The model under review builds one solid part; all positions refer to its coordinate system, in mm. A direction names the side the tool comes from. Give positions to 0.01 mm unless a question says otherwise; leave off trailing zeros. Loops run counter-clockwise (first coordinate to the right, second up) from the corner with the lowest first, then second, coordinate; pieces in that order, holes last. Notation, with made-up numbers: M 88.25,16.25 L 115.25,16.25 A21 ccw 115.25,36.25 Z; hole C 62.5,-14.5 d5. An arc over 180 degrees is marked long. Put each result on its own line as item: value. Start each with the question number.
```python
from build123d import *

# Parameters (mm, degrees)
SKETCH_1_R               = 6
SKETCH_1_R_2             = 4
EXTRUDE_1_DEPTH          = 5
CUT_EXTRUDE_1_REACH      = 16.318
CUT_EXTRUDE_1_END_RADIUS = 4
SKETCH_2_R               = 1.45
SKETCH_3_W               = 30
SKETCH_3_H               = 31
SKETCH_3_R               = 6
EXTRUDE_1_2_DEPTH        = 2
SKETCH_6_W               = 2
SKETCH_6_H               = 4
EXTRUDE_2_DEPTH          = 12
EXTRUDE_3_DEPTH          = 1.5
EXTRUDE_START            = -1.25
EXTRUDE_4_DEPTH          = 1.5
CUT_EXTRUDE_3_REACH      = 30.745
SKETCH_11_R              = 0.95
CUT_EXTRUDE_4_REACH      = 30.745
SKETCH_12_R              = 0.95
CUT_EXTRUDE_5_REACH      = 26.683
SKETCH_14_W              = 2
SKETCH_14_H              = 12
CUT_EXTRUDE_6_DEPTH      = 0.3
SKETCH_15_W              = 2
SKETCH_15_H              = 12
CUT_EXTRUDE_7_DEPTH      = 0.3


with BuildPart() as part:
    # 草图1 → Extrude 1 (new body)
    with BuildSketch(Plane(origin=(0, 0, 0), x_dir=(1, 0, 0), z_dir=(0, 1, 0))):
        Circle(SKETCH_1_R)
        Circle(SKETCH_1_R_2, mode=Mode.SUBTRACT)
    extrude(amount=EXTRUDE_1_DEPTH)

    # 切除-拉伸1: up to this cylinder (the profile starts outside it)
    cut_extrude_1_end = Plane(origin=(0, 2.637062, 0), z_dir=(0, -1, 0)) * Cylinder(CUT_EXTRUDE_1_END_RADIUS, 41.636, mode=Mode.PRIVATE)
    # 草图2 → 切除-拉伸1 (cut, up to the surface)
    with BuildSketch(Plane(origin=(6, 0, 0), x_dir=(0, 0, -1), z_dir=(1, 0, 0)), mode=Mode.PRIVATE) as cut_extrude_1_sk1:
        with Locations((0, 2.637062232)):
            Circle(SKETCH_2_R)
    cut_extrude_1_tool1 = extrude(cut_extrude_1_sk1.sketch, amount=-CUT_EXTRUDE_1_REACH, mode=Mode.PRIVATE) - cut_extrude_1_end
    add(cut_extrude_1_tool1.solids().sort_by_distance((6, 2.637062, 0))[0], mode=Mode.SUBTRACT)

    # 草图3 → Extrude 1 2 (add)
    # profile 1 of 2: a face of its own
    with BuildSketch(Plane(origin=(0, 5, 0), x_dir=(1, 0, 0), z_dir=(0, 1, 0))):
        Rectangle(SKETCH_3_W, SKETCH_3_H)
        Circle(SKETCH_3_R, mode=Mode.SUBTRACT)
    # profile 2 of 2: a face of its own
    with BuildSketch(Plane(origin=(0, 5, 0), x_dir=(1, 0, 0), z_dir=(0, 1, 0))):
        Circle(SKETCH_3_R)
    extrude(amount=EXTRUDE_1_2_DEPTH)

    # 草图6 → 凸台-拉伸2 (add)
    with BuildSketch(Plane(origin=(0, 7, 0), x_dir=(1, 0, 0), z_dir=(0, 1, 0))):
        with Locations((-1, 13.5)):
            Rectangle(SKETCH_6_W, SKETCH_6_H)
        with Locations((-1, -13.5)):
            Rectangle(SKETCH_6_W, SKETCH_6_H)
    extrude(amount=EXTRUDE_2_DEPTH)

    # 草图9 → 凸台-拉伸3 (add)
    with BuildSketch(Plane.XY.offset(-12.75)):
        Polygon((-2, 7), (-8, 7), (-2, 17), align=None)
    extrude(amount=-EXTRUDE_3_DEPTH)

    # 草图10 → 凸台-拉伸4 (add)
    with BuildSketch(Plane.XY.offset(15.5).offset(EXTRUDE_START)):
        Polygon((-2, 7), (-2, 17), (-8, 7), align=None)
    extrude(amount=-EXTRUDE_4_DEPTH)

    # 草图11 → 切除-拉伸3 (cut, up to next)
    with BuildSketch(Plane(origin=(0, 0, 0), x_dir=(0, 0, -1), z_dir=(1, 0, 0)), mode=Mode.PRIVATE) as cut_extrude_3_sk1:
        with Locations((-13.5, 13)):
            Circle(SKETCH_11_R)
    cut_extrude_3_tool1 = extrude(cut_extrude_3_sk1.sketch, amount=-CUT_EXTRUDE_3_REACH, mode=Mode.PRIVATE) & part.part
    add(cut_extrude_3_tool1.solids().sort_by_distance((0, 13, 13.5))[0], mode=Mode.SUBTRACT)

    # 草图12 → 切除-拉伸4 (cut, up to next)
    with BuildSketch(Plane(origin=(0, 0, 0), x_dir=(0, 0, -1), z_dir=(1, 0, 0)), mode=Mode.PRIVATE) as cut_extrude_4_sk1:
        with Locations((13.5, 13)):
            Circle(SKETCH_12_R)
    cut_extrude_4_tool1 = extrude(cut_extrude_4_sk1.sketch, amount=-CUT_EXTRUDE_4_REACH, mode=Mode.PRIVATE) & part.part
    add(cut_extrude_4_tool1.solids().sort_by_distance((0, 13, -13.5))[0], mode=Mode.SUBTRACT)

    # 草图13 → 切除-拉伸5 (cut, up to next)
    with BuildSketch(Plane(origin=(0, 7, 0), x_dir=(1, 0, 0), z_dir=(0, 1, 0)), mode=Mode.PRIVATE) as cut_extrude_5_sk1:
        with BuildLine():
            ThreePointArc((-5.178078794, -15.5), (-6.61861505, -14.941768129), (-8, -14.25))
            ThreePointArc((-8, -14.25), (-12.137612149, -10.942617206), (-15, -6.485560886))
            Line((-15, -6.485560886), (-15, -15.5))
            Line((-15, -15.5), (-5.178078794, -15.5))
        make_face()
    cut_extrude_5_tool1 = extrude(cut_extrude_5_sk1.sketch, amount=-CUT_EXTRUDE_5_REACH, mode=Mode.PRIVATE) & part.part
    # 草图13 → 切除-拉伸5 (cut, up to next)
    with BuildSketch(Plane(origin=(0, 7, 0), x_dir=(1, 0, 0), z_dir=(0, 1, 0)), mode=Mode.PRIVATE) as cut_extrude_5_sk2:
        with BuildLine():
            ThreePointArc((15, -6.485560886), (11.050056294, -12.039881889), (5.178078794, -15.5))
            Line((5.178078794, -15.5), (15, -15.5))
            Line((15, -15.5), (15, -6.485560886))
        make_face()
    cut_extrude_5_tool2 = extrude(cut_extrude_5_sk2.sketch, amount=-CUT_EXTRUDE_5_REACH, mode=Mode.PRIVATE) & part.part
    # 草图13 → 切除-拉伸5 (cut, up to next)
    with BuildSketch(Plane(origin=(0, 7, 0), x_dir=(1, 0, 0), z_dir=(0, 1, 0)), mode=Mode.PRIVATE) as cut_extrude_5_sk3:
        with BuildLine():
            ThreePointArc((5.178078794, 15.5), (11.050056294, 12.039881889), (15, 6.485560886))
            Line((15, 6.485560886), (15, 15.5))
            Line((15, 15.5), (5.178078794, 15.5))
        make_face()
    cut_extrude_5_tool3 = extrude(cut_extrude_5_sk3.sketch, amount=-CUT_EXTRUDE_5_REACH, mode=Mode.PRIVATE) & part.part
    # 草图13 → 切除-拉伸5 (cut, up to next)
    with BuildSketch(Plane(origin=(0, 7, 0), x_dir=(1, 0, 0), z_dir=(0, 1, 0)), mode=Mode.PRIVATE) as cut_extrude_5_sk4:
        with BuildLine():
            Line((-15, 15.5), (-15, 6.485560886))
            ThreePointArc((-15, 6.485560886), (-12.137612149, 10.942617206), (-8, 14.25))
            ThreePointArc((-8, 14.25), (-6.61861505, 14.941768129), (-5.178078794, 15.5))
            Line((-5.178078794, 15.5), (-15, 15.5))
        make_face()
    cut_extrude_5_tool4 = extrude(cut_extrude_5_sk4.sketch, amount=-CUT_EXTRUDE_5_REACH, mode=Mode.PRIVATE) & part.part
    add(cut_extrude_5_tool1.solids().sort_by_distance((-12.231882, 7, 12.932652))[0], mode=Mode.SUBTRACT)
    add(cut_extrude_5_tool2.solids().sort_by_distance((12.231882, 7, 12.932652))[0], mode=Mode.SUBTRACT)
    add(cut_extrude_5_tool3.solids().sort_by_distance((12.231882, 7, -12.932652))[0], mode=Mode.SUBTRACT)
    add(cut_extrude_5_tool4.solids().sort_by_distance((-12.231882, 7, -12.932652))[0], mode=Mode.SUBTRACT)

    # 草图14 → 切除-拉伸6 (cut)
    with BuildSketch(Plane(origin=(0, 0, 11.5), x_dir=(-1, 0, 0), z_dir=(0, 0, -1))):
        with Locations((1, 13)):
            Rectangle(SKETCH_14_W, SKETCH_14_H)
    extrude(amount=-CUT_EXTRUDE_6_DEPTH, mode=Mode.SUBTRACT)

    # 草图15 → 切除-拉伸7 (cut)
    with BuildSketch(Plane.XY.offset(-11.5)):
        with Locations((-1, 13)):
            Rectangle(SKETCH_15_W, SKETCH_15_H)
    extrude(amount=-CUT_EXTRUDE_7_DEPTH, mode=Mode.SUBTRACT)


solid = part.part
```
Item 1: Tool access review of faces 4 (the flat face through (-4, 7, -15)), 5 (the flat face through (0, 13, 15)), 6 (the flat face through (-4, 9, 12.75)), 7 (the flat face through (-4, 9, 14.25)): name each direction out of +Z, -Z, +X, -X, +Y, -Y from which nothing blocks a thin tool from reaching the whole face with its end or side.
Item 2: Draft analysis for pull direction Z (two halves, no side actions). For faces 1 (the flat face through (15, 6, 0)), 2 (the flat face through (-3, 15, -14.25)), 3 (the flat face through (-1, 13, 11.8)), state which applies: +Z half, -Z half, draft (parallel to the pull), parting line (faces both ways), or undercut.
Item 3: Consider section C-C, the plane x = 0.75. Write out the cut boundary in (y, z), plus the area to 3 significant figures.
Item 4: Consider section D-D, the plane z = -5. Write out the cut boundary in (x, y), plus the area to 3 significant figures.
Item 5: Consider section A-A, the plane y = 15.5. Write out the cut boundary in (x, z).
Item 6: To check wall thickness, follow L1, parallel to Z at x = -1, y = 13; L2, parallel to Y at x = -3.2, z = -13.5; L3, parallel to Y at x = -2.9, z = -13.5. State the ranges of each line that lie inside material, in increasing order. Write a range as [from, to].
Item 7: Clearance check with flat-ended pins moving along their axes: pin 1 Ø1 at (x, y) = (-3, 15) entering from +Z; pin 2 Ø3 at (y, z) = (13.5, -14) entering from +X; pin 3 Ø4.5 at (x, y) = (-4.5, 9.5) entering from +Z; pin 4 Ø1 at (x, y) = (-3.5, 16.5) entering from +Z. State where each tip first meets the part, or that it passes through.
Item 8: Consider section B-B, the plane z = 0. Write out the cut boundary in (x, y).
Report:
1. face 4: -Z, -X, +Y
1. face 5: +Z, -Z, +X, +Y
1. face 6: -X, +Y
1. face 7: +Z, -X, +Y
2. face 1: draft
2. face 2: -Z half
2. face 3: undercut
3. outline: M 0,-5.95 L 5,-5.95 L 5,-15.5 L 7,-15.5 L 7,15.5 L 5,15.5 L 5,5.95 L 0,5.95 L 0,3.93 L 5,3.93 L 5,-3.93 L 0,-3.93 Z
3. area: 82.2 mm²
4. outline: M -15,5 L -3.32,5 L -3.32,0 L 3.32,0 L 3.32,5 L 15,5 L 15,7 L -15,7 Z
4. area: 93.2 mm²
5. outline: M -2.9,-14.25 L -2,-14.25 L -2,-15.5 L 0,-15.5 L 0,-11.8 L -2,-11.8 L -2,-12.75 L -2.9,-12.75 Z; M -2.9,12.75 L -2,12.75 L -2,11.8 L 0,11.8 L 0,15.5 L -2,15.5 L -2,14.25 L -2.9,14.25 Z
6. L1: [-15.5, -14.45], [-12.55, -11.8], [11.8, 12.55], [14.45, 15.5]
6. L2: [5, 12.05], [13.95, 15]
6. L3: [5, 12.05], [13.95, 15.5]
7. pin 1: z = 14.25
7. pin 2: x = 0
7. pin 3: z = 14.25
7. pin 4: through
8. outline: M -15,5 L -6,5 L -6,0 L -4,0 L -4,5 L 4,5 L 4,4.09 L 6,4.09 L 6,5 L 15,5 L 15,7 L -15,7 Z; M 4,0 L 6,0 L 6,1.19 L 4,1.19 Z
